Verification items for the finished model (mm, model axes). Face numbers are marked on the shaded views. A direction names the side the tool comes from. Give positions to 0.01 mm unless a question says otherwise; leave off trailing zeros. Write each loop counter-clockwise with the first axis right and the second up, starting at its lowest first coordinate (ties: lowest second). Pieces come first, ordered by that corner, then holes. Notation, with made-up numbers: (-19.5, 78.5) -> (35.5, 78.5) arc R25 ccw to (35.5, 99.5) -> close; hole circle Ø4 at (20.25, 63.5). An arc over 180 degrees is marked (long way). Use one line per item in the form item = value. Start each with the question number.
(1) Section check A-A, the plane y = -2. Record the cut outline in (x, z).
(2) Scan lines: L1, parallel to Z at x = 52, y = -12; L2, parallel to X at y = 14.5, z = 39; L3, parallel to Y at x = 59, z = 62. Record each from-to range of solid material in increasing order.
(3) Release check for a two-part mould opening along X. For the marked faces 3, 4, 5 and 6 record: pulls with the +X half, pulls with the -X half, needs draft (parallel to the pull), parting line crosses it, or undercut.
(4) Section check B-B, the plane z = 37. Record the cut outline in (x, y).
(5) Section check C-C, the plane x = 44. Record the cut outline in (y, z), plus the area to 3 significant figures.
(6) Depth check by flat-ended pin: pin 1 Ø1 at (x, z) = (-4.5, 67) entering from +Y; pin 2 Ø1.5 at (y, z) = (-13.5, 18.5) entering from +X. Enter the tip coordinate at first touch or a pass-through.
(7) Set-up check for the marked faces 1 and 2: record each of +Z, -Z, +X, -X, +Y, -Y from which the full face is reachable in a straight line by a thin tool's end or side.
(8) Section check D-D, the plane z = 70. Record the cut outline in (x, y).
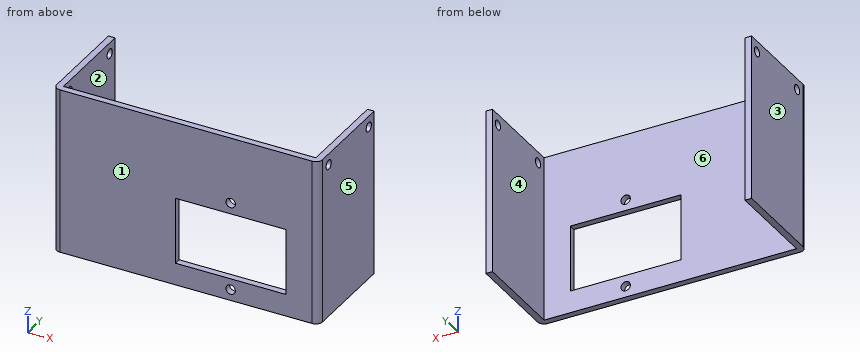
from build123d import *

# Parameters (mm, degrees)
F1_DEPTH = 75
F2_R     = 2.125
F2_W     = 50
F2_H     = 30
F3_DEPTH = 5
F5_R     = 2.125
F6_DEPTH = 130
F7_R     = 3


with BuildPart() as f1:
    # F0 (on Top) → F1 (new body)
    with BuildSketch(Plane.XY):
        Polygon((-28.58369, -11.800445), (-28.58369, 30.699555), (-30.356892, 30.699555), (-31.58369, 30.699555), (-31.58369, -14.800445), (-27.58369, -14.800445), (84.41631, -14.800445), (88.41631, -14.800445), (88.41631, 30.699555), (87.189512, 30.699555), (85.41631, 30.699555), (85.41631, -11.800445), align=None)
    extrude(amount=F1_DEPTH)

    # F2 (on face) → F3 (cut)
    with BuildSketch(Plane.XZ.offset(14.800445)):
        with Locations((48.598289, 45)):
            Circle(F2_R)
        with Locations((48.598289, 5)):
            Circle(F2_R)
        with Locations((48.598289, 25)):
            Rectangle(F2_W, F2_H)
    extrude(amount=-F3_DEPTH, mode=Mode.SUBTRACT)

    # F5 (on face) → F6 (cut)
    with BuildSketch(Plane.YZ.offset(88.41631)):
        with Locations((-6.730337, 70)):
            Circle(F5_R)
        with Locations((26.269663, 70)):
            Circle(F5_R)
    extrude(amount=-F6_DEPTH, mode=Mode.SUBTRACT)

    # F7
    f7_edges = [f1.edges().sort_by_distance(p)[0] for p in [
        (88.41631, -14.800445, 37.5),
        (-31.58369, -14.800445, 37.5),
    ]]
    fillet(f7_edges, radius=F7_R)


solid = f1.part
Completed:
q1.outline = (-31.58, 0) -> (-28.58, 0) -> (-28.58, 75) -> (-31.58, 75) -> close; (85.42, 0) -> (88.42, 0) -> (88.42, 75) -> (85.42, 75) -> close
q2.L1 = 0 to 10, 40 to 75
q2.L2 = -31.58 to -28.58, 85.42 to 88.42
q2.L3 = -14.8 to -11.8
q3.face_3 = pulls with the -X half
q3.face_4 = undercut
q3.face_5 = pulls with the +X half
q3.face_6 = undercut
q4.outline = (-31.58, -11.8) arc R3 ccw to (-28.58, -14.8) -> (23.6, -14.8) -> (23.6, -11.8) -> (-28.58, -11.8) -> (-28.58, 30.7) -> (-31.58, 30.7) -> close; (73.6, -14.8) -> (85.42, -14.8) arc R3 ccw to (88.42, -11.8) -> (88.42, 30.7) -> (85.42, 30.7) -> (85.42, -11.8) -> (73.6, -11.8) -> close
q5.outline = (-14.8, 0) -> (-11.8, 0) -> (-11.8, 10) -> (-14.8, 10) -> close; (-14.8, 40) -> (-11.8, 40) -> (-11.8, 75) -> (-14.8, 75) -> close
q5.area = 135 mm²
q6.pin_1 = -11.8
q6.pin_2 = 88.26
q7.face_1 = +Z, -Z, +X, -X, -Y
q7.face_2 = +Z, -Z, +Y
q8.outline = (-31.58, -11.8) arc R3 ccw to (-28.58, -14.8) -> (85.42, -14.8) arc R3 ccw to (88.42, -11.8) -> (88.42, -8.86) -> (85.42, -8.86) -> (85.42, -11.8) -> (-28.58, -11.8) -> (-28.58, -8.86) -> (-31.58, -8.86) -> close; (-31.58, -4.61) -> (-28.58, -4.61) -> (-28.58, 24.14) -> (-31.58, 24.14) -> close; (-31.58, 28.39) -> (-28.58, 28.39) -> (-28.58, 30.7) -> (-31.58, 30.7) -> close; (85.42, -4.61) -> (88.42, -4.61) -> (88.42, 24.14) -> (85.42, 24.14) -> close; (85.42, 28.39) -> (88.42, 28.39) -> (88.42, 30.7) -> (85.42, 30.7) -> close
